The drawing under review shows one solid part. Ordinate dimensions are in mm from its lowest x, y, z. A direction names the side the tool comes from. Give positions to 0.01 mm unless a question says otherwise; leave off trailing zeros. Order: outer loops, then holes, each group sorted by start corner. A loop starts at its lowest first (then second) coordinate and runs counter-clockwise, first axis right, second up. Notation, with made-up numbers: (64.5, -6.5) - (82.5, -6.5) arc R22 cw to (82.5, 25.5) - close; hole circle Ø5 at (59, 64.5). An arc over 180 degrees is marked (long way). Write item = value, one per line. Start each with the question number.
1. We need section C-C, the plane x = 27.5. Give the boundary of the cut face in (y, z) (1 decimal).
2. We need section B-B, the plane y = 16. Give the boundary of the cut face in (x, z), and give its area (3 significant figures).
3. Machinability: for the marked faces 4 and 5, which of the approach directions +Z, -Z, +X, -X, +Y, -Y give a long, thin tool a straight path to every point of the face, cutting with its end or side? Answer none if there is none.
4. Mouldability with a two-part tool opening along X and no side actions: class the marked faces 1, 2 and 3 as pulls with the +X half, pulls with the -X half, needs draft (parallel to the pull), parting line crosses it, or undercut.
5. We need section D-D, the plane z = 17. Give the boundary of the cut face in (x, y) (1 decimal).
6. Wall thickness on probe 1 along Y at (x, z) = (4, 20.5) (1 decimal); probe 2 along Z at (x, y) = (31.5, 28.5); probe 3 along X at (y, z) = (13.5, 39.5) (1 decimal): over which ranges is each line inside the solid? List them lowest first.
7. For P1, Ø11.5, axis at x = 19.15, z = 36.58, coming from the +Y side (1 decimal); P2, Ø5, axis at x = 23.5, y = 12, coming from the -Z side; P3, Ø6, axis at x = 29, y = 29, coming from the +Z side, all flat-tipped, find the tip position at first contact; note any pin that passes through.
8. We need section A-A, the plane x = 17. Give the boundary of the cut face in (y, z) (1 decimal), and give its area (3 significant figures).
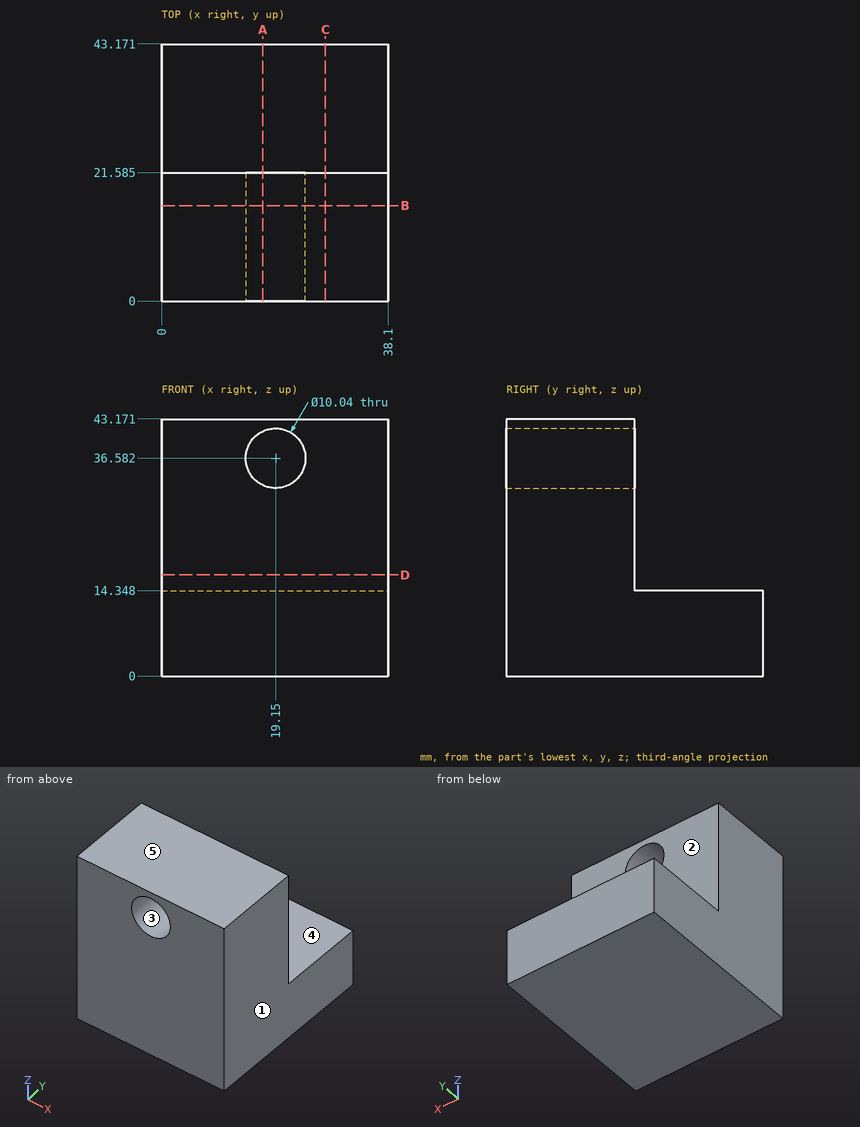
Model answer:
q1.outline = (0, 0) - (43.2, 0) - (43.2, 14.3) - (21.6, 14.3) - (21.6, 43.2) - (0, 43.2) - close
q2.outline = (0, 0) - (38.1, 0) - (38.1, 43.17) - (0, 43.17) - close; hole circle Ø10.04 at (19.15, 36.58)
q2.area = 1,570 mm2
q3.face_4 = +Z, +X, -X, +Y
q3.face_5 = +Z, +X, -X, +Y, -Y
q4.face_1 = pulls with the +X half
q4.face_2 = needs draft
q4.face_3 = undercut
q5.outline = (0, 0) - (38.1, 0) - (38.1, 21.6) - (0, 21.6) - close
q6.probe_1 = 0 to 21.6
q6.probe_2 = 0 to 14.35
q6.probe_3 = 0 to 15.1, 23.2 to 38.1
q7.P1 = 21.6
q7.P2 = 0
q7.P3 = 14.35
q8.outline = (0, 0) - (43.2, 0) - (43.2, 14.3) - (21.6, 14.3) - (21.6, 32) - (0, 32) - close; (0, 41.1) - (21.6, 41.1) - (21.6, 43.2) - (0, 43.2) - close
q8.area = 1,050 mm2
